```python
from build123d import *

# Parameters (mm, degrees)
BOSS_EXTRUDE1_DEPTH      = 20
BOSS_EXTRUDE1_DEPTH_BACK = 20
SKETCH1_W                = 35
SKETCH1_H                = 85.2
CUT_EXTRUDE2_REACH       = 91.478
SKETCH5_R                = 1.55
SKETCH5_R_2              = 2.9
CUT_EXTRUDE3_DEPTH       = 8
BOSS_EXTRUDE2_DEPTH      = 40


with BuildPart() as part:
    # Sketch1 → Boss-Extrude1 (new, two sides: drawn at the far end of the back side and taken through both)
    with BuildSketch(Plane.XY.offset(-BOSS_EXTRUDE1_DEPTH_BACK)):
        with Locations((1.938408795, -35.043181818)):
            Rectangle(SKETCH1_W, SKETCH1_H)
    extrude(amount=BOSS_EXTRUDE1_DEPTH + BOSS_EXTRUDE1_DEPTH_BACK)

    # Sketch2 → Cut-Extrude2 (cut, up to next)
    with BuildSketch(Plane.XY.offset(20), mode=Mode.PRIVATE) as cut_extrude2_sk1:
        with BuildLine():
            Line((-9.561591205, -10.793181818), (-9.561591205, -15.293181818))
            ThreePointArc((-9.561591205, -15.293181818), (-9.268697986, -16.000288599), (-8.561591205, -16.293181818))
            Line((-8.561591205, -16.293181818), (12.438408795, -16.293181818))
            ThreePointArc((12.438408795, -16.293181818), (13.145515577, -16.000288599), (13.438408795, -15.293181818))
            Line((13.438408795, -15.293181818), (13.438408795, -10.793181818))
            ThreePointArc((13.438408795, -10.793181818), (13.145515577, -10.086075037), (12.438408795, -9.793181818))
            Line((12.438408795, -9.793181818), (-8.561591205, -9.793181818))
            ThreePointArc((-8.561591205, -9.793181818), (-9.268697986, -10.086075037), (-9.561591205, -10.793181818))
        make_face()
    cut_extrude2_tool1 = extrude(cut_extrude2_sk1.sketch, amount=-CUT_EXTRUDE2_REACH, mode=Mode.PRIVATE) & part.part
    # Sketch2 → Cut-Extrude2 (cut, up to next)
    with BuildSketch(Plane.XY.offset(20), mode=Mode.PRIVATE) as cut_extrude2_sk2:
        with BuildLine():
            Line((-9.561591205, -21.793181818), (-9.561591205, -26.293181818))
            ThreePointArc((-9.561591205, -26.293181818), (-9.268697986, -27.000288599), (-8.561591205, -27.293181818))
            Line((-8.561591205, -27.293181818), (12.438408795, -27.293181818))
            ThreePointArc((12.438408795, -27.293181818), (13.145515577, -27.000288599), (13.438408795, -26.293181818))
            Line((13.438408795, -26.293181818), (13.438408795, -21.793181818))
            ThreePointArc((13.438408795, -21.793181818), (13.145515577, -21.086075037), (12.438408795, -20.793181818))
            Line((12.438408795, -20.793181818), (-8.561591205, -20.793181818))
            ThreePointArc((-8.561591205, -20.793181818), (-9.268697986, -21.086075037), (-9.561591205, -21.793181818))
        make_face()
    cut_extrude2_tool2 = extrude(cut_extrude2_sk2.sketch, amount=-CUT_EXTRUDE2_REACH, mode=Mode.PRIVATE) & part.part
    # Sketch2 → Cut-Extrude2 (cut, up to next)
    with BuildSketch(Plane.XY.offset(20), mode=Mode.PRIVATE) as cut_extrude2_sk3:
        with BuildLine():
            Line((-8.561591205, 1.206818182), (12.438408795, 1.206818182))
            ThreePointArc((12.438408795, 1.206818182), (13.145515577, 0.913924963), (13.438408795, 0.206818182))
            Line((13.438408795, 0.206818182), (13.438408795, -4.293181818))
            ThreePointArc((13.438408795, -4.293181818), (13.145515577, -5.000288599), (12.438408795, -5.293181818))
            Line((12.438408795, -5.293181818), (-8.561591205, -5.293181818))
            ThreePointArc((-8.561591205, -5.293181818), (-9.268697986, -5.000288599), (-9.561591205, -4.293181818))
            Line((-9.561591205, -4.293181818), (-9.561591205, 0.206818182))
            ThreePointArc((-9.561591205, 0.206818182), (-9.268697986, 0.913924963), (-8.561591205, 1.206818182))
        make_face()
    cut_extrude2_tool3 = extrude(cut_extrude2_sk3.sketch, amount=-CUT_EXTRUDE2_REACH, mode=Mode.PRIVATE) & part.part
    # Sketch2 → Cut-Extrude2 (cut, up to next)
    with BuildSketch(Plane.XY.offset(20), mode=Mode.PRIVATE) as cut_extrude2_sk4:
        with BuildLine():
            Line((-9.561591205, -32.793181818), (-9.561591205, -37.293181818))
            ThreePointArc((-9.561591205, -37.293181818), (-9.268697986, -38.000288599), (-8.561591205, -38.293181818))
            Line((-8.561591205, -38.293181818), (12.438408795, -38.293181818))
            ThreePointArc((12.438408795, -38.293181818), (13.145515577, -38.000288599), (13.438408795, -37.293181818))
            Line((13.438408795, -37.293181818), (13.438408795, -32.793181818))
            ThreePointArc((13.438408795, -32.793181818), (13.145515577, -32.086075037), (12.438408795, -31.793181818))
            Line((12.438408795, -31.793181818), (-8.561591205, -31.793181818))
            ThreePointArc((-8.561591205, -31.793181818), (-9.268697986, -32.086075037), (-9.561591205, -32.793181818))
        make_face()
    cut_extrude2_tool4 = extrude(cut_extrude2_sk4.sketch, amount=-CUT_EXTRUDE2_REACH, mode=Mode.PRIVATE) & part.part
    # Sketch2 → Cut-Extrude2 (cut, up to next)
    with BuildSketch(Plane.XY.offset(20), mode=Mode.PRIVATE) as cut_extrude2_sk5:
        with BuildLine():
            Line((-9.561591205, -43.793181818), (-9.561591205, -48.293181818))
            ThreePointArc((-9.561591205, -48.293181818), (-9.268697986, -49.000288599), (-8.561591205, -49.293181818))
            Line((-8.561591205, -49.293181818), (12.438408795, -49.293181818))
            ThreePointArc((12.438408795, -49.293181818), (13.145515577, -49.000288599), (13.438408795, -48.293181818))
            Line((13.438408795, -48.293181818), (13.438408795, -43.793181818))
            ThreePointArc((13.438408795, -43.793181818), (13.145515577, -43.086075037), (12.438408795, -42.793181818))
            Line((12.438408795, -42.793181818), (-8.561591205, -42.793181818))
            ThreePointArc((-8.561591205, -42.793181818), (-9.268697986, -43.086075037), (-9.561591205, -43.793181818))
        make_face()
    cut_extrude2_tool5 = extrude(cut_extrude2_sk5.sketch, amount=-CUT_EXTRUDE2_REACH, mode=Mode.PRIVATE) & part.part
    # Sketch2 → Cut-Extrude2 (cut, up to next)
    with BuildSketch(Plane.XY.offset(20), mode=Mode.PRIVATE) as cut_extrude2_sk6:
        with BuildLine():
            Line((-9.561591205, -54.793181818), (-9.561591205, -59.293181818))
            ThreePointArc((-9.561591205, -59.293181818), (-9.268697986, -60.000288599), (-8.561591205, -60.293181818))
            Line((-8.561591205, -60.293181818), (12.438408795, -60.293181818))
            ThreePointArc((12.438408795, -60.293181818), (13.145515577, -60.000288599), (13.438408795, -59.293181818))
            Line((13.438408795, -59.293181818), (13.438408795, -54.793181818))
            ThreePointArc((13.438408795, -54.793181818), (13.145515577, -54.086075037), (12.438408795, -53.793181818))
            Line((12.438408795, -53.793181818), (-8.561591205, -53.793181818))
            ThreePointArc((-8.561591205, -53.793181818), (-9.268697986, -54.086075037), (-9.561591205, -54.793181818))
        make_face()
    cut_extrude2_tool6 = extrude(cut_extrude2_sk6.sketch, amount=-CUT_EXTRUDE2_REACH, mode=Mode.PRIVATE) & part.part
    # Sketch2 → Cut-Extrude2 (cut, up to next)
    with BuildSketch(Plane.XY.offset(20), mode=Mode.PRIVATE) as cut_extrude2_sk7:
        with BuildLine():
            Line((-9.561591205, -65.793181818), (-9.561591205, -70.293181818))
            ThreePointArc((-9.561591205, -70.293181818), (-9.268697986, -71.000288599), (-8.561591205, -71.293181818))
            Line((-8.561591205, -71.293181818), (12.438408795, -71.293181818))
            ThreePointArc((12.438408795, -71.293181818), (13.145515577, -71.000288599), (13.438408795, -70.293181818))
            Line((13.438408795, -70.293181818), (13.438408795, -65.793181818))
            ThreePointArc((13.438408795, -65.793181818), (13.145515577, -65.086075037), (12.438408795, -64.793181818))
            Line((12.438408795, -64.793181818), (-8.561591205, -64.793181818))
            ThreePointArc((-8.561591205, -64.793181818), (-9.268697986, -65.086075037), (-9.561591205, -65.793181818))
        make_face()
    cut_extrude2_tool7 = extrude(cut_extrude2_sk7.sketch, amount=-CUT_EXTRUDE2_REACH, mode=Mode.PRIVATE) & part.part
    add(cut_extrude2_tool1.solids().sort_by_distance((1.938409, -13.043182, 20))[0], mode=Mode.SUBTRACT)
    add(cut_extrude2_tool2.solids().sort_by_distance((1.938409, -24.043182, 20))[0], mode=Mode.SUBTRACT)
    add(cut_extrude2_tool3.solids().sort_by_distance((1.938409, -2.043182, 20))[0], mode=Mode.SUBTRACT)
    add(cut_extrude2_tool4.solids().sort_by_distance((1.938409, -35.043182, 20))[0], mode=Mode.SUBTRACT)
    add(cut_extrude2_tool5.solids().sort_by_distance((1.938409, -46.043182, 20))[0], mode=Mode.SUBTRACT)
    add(cut_extrude2_tool6.solids().sort_by_distance((1.938409, -57.043182, 20))[0], mode=Mode.SUBTRACT)
    add(cut_extrude2_tool7.solids().sort_by_distance((1.938409, -68.043182, 20))[0], mode=Mode.SUBTRACT)

    # Sketch5 → Cut-Extrude3 (cut)
    with BuildSketch(Plane(origin=(0, 7.556818182, 0), x_dir=(1, 0, 0), z_dir=(0, 1, 0))):
        with Locations(Location((-3.046694012, 4.985102807, 0), (0, 0, 270))):
            Circle(SKETCH5_R)
        with Locations(Location((1.938408795, 0, 0), (0, 0, 270))):
            Circle(SKETCH5_R_2)
        with Locations(Location((6.923511603, 4.985102807, 0), (0, 0, 270))):
            Circle(SKETCH5_R)
        with Locations(Location((6.923511603, -4.985102807, 0), (0, 0, 270))):
            Circle(SKETCH5_R)
        with Locations(Location((-3.046694012, -4.985102807, 0), (0, 0, 270))):
            Circle(SKETCH5_R)
    cut_extrude3 = extrude(amount=-CUT_EXTRUDE3_DEPTH, mode=Mode.SUBTRACT)

    # Mirror3: Cut-Extrude3 across plane
    add(cut_extrude3.mirror(Plane.ZX.offset(-35.043181818)), mode=Mode.SUBTRACT)

    # Sketch7 → Boss-Extrude2 (add)
    with BuildSketch(Plane(origin=(0, 0, -20), x_dir=(-1, 0, 0), z_dir=(0, 0, -1))):
        with BuildLine():
            Line((-19.438408795, 7.556818182), (-21.818320385, 7.556818182))
            ThreePointArc((-21.818320385, 7.556818182), (-23.528170709, 6.594320889), (-23.592294725, 4.633230049))
            Line((-23.592294725, 4.633230049), (-20.794562752, -0.740490723))
            ThreePointArc((-20.794562752, -0.740490723), (-19.782377041, -3.429490161), (-19.438408795, -6.282019519))
            Line((-19.438408795, -6.282019519), (-19.438408795, 7.556818182))
        make_face()
        with BuildLine():
            Line((15.561591205, -77.643181818), (17.941502794, -77.643181818))
            ThreePointArc((17.941502794, -77.643181818), (19.651353118, -76.680684525), (19.715477134, -74.719593686))
            Line((19.715477134, -74.719593686), (16.917745161, -69.345872913))
            ThreePointArc((16.917745161, -69.345872913), (15.90555945, -66.656873475), (15.561591205, -63.804344117))
            Line((15.561591205, -63.804344117), (15.561591205, -77.643181818))
        make_face()
        with BuildLine():
            Line((-19.438408795, -63.804344117), (-19.438408795, -77.643181818))
            Line((-19.438408795, -77.643181818), (-21.818320385, -77.643181818))
            ThreePointArc((-21.818320385, -77.643181818), (-23.528170709, -76.680684525), (-23.592294725, -74.719593686))
            Line((-23.592294725, -74.719593686), (-20.794562752, -69.345872913))
            ThreePointArc((-20.794562752, -69.345872913), (-19.782377041, -66.656873475), (-19.438408795, -63.804344117))
        make_face()
        with BuildLine():
            Line((15.561591205, -6.282019519), (15.561591205, 7.556818182))
            Line((15.561591205, 7.556818182), (17.941502794, 7.556818182))
            ThreePointArc((17.941502794, 7.556818182), (19.651353118, 6.594320889), (19.715477134, 4.633230049))
            Line((19.715477134, 4.633230049), (16.917745161, -0.740490723))
            ThreePointArc((16.917745161, -0.740490723), (15.90555945, -3.429490161), (15.561591205, -6.282019519))
        make_face()
    extrude(amount=-BOSS_EXTRUDE2_DEPTH)


solid = part.part
```
Model file for the job. Use its own axes, mm. A direction names the side the tool comes from. Coordinates: 2 decimals unless noted, no trailing zeros. Order: outer loops, then holes, each group sorted by start corner. A loop starts at its lowest first (then second) coordinate and runs counter-clockwise, first axis right, second up. Notation, with made-up numbers: (44, 49.25) -> (74, 49.25) arc R21 cw to (74, 82.25) -> close; hole circle Ø10 at (-36, 57.5). An arc over 180 degrees is marked (long way). Return JSON: item names as keys, results as strings.
Item 1: 3-axis set-ups, long thin cutter, end or side, ignore diameter. For faces 1 (the face through (-15.915, -3.39, -0.28)), 2 (the face through (7.389, -74.513, 6.464)), 3 (the face through (-9.562, -35, 0)), 4 (the face through (7.389, 4.426, 6.464)): which of +Z, -Z, +X, -X, +Y, -Y reach the whole face in a straight line?
Model answer:
{"face 1": "+Z, -Z, -X", "face 2": "-Y", "face 3": "+Z, -Z", "face 4": "+Y"}
Item 2: Mould opens along X. For faces 5 (the face through (-15.915, -66.696, -0.28)), 6 (the face through (-9.562, -46, 0)), 7 (the face through (23.51, -76.71, -0.28)) say: pulls with the +X half, pulls with the -X half, needs draft (parallel to the pull), parting line crosses it, or undercut.
Model answer:
{"face 5": "pulls with the -X half", "face 6": "undercut", "face 7": "pulls with the +X half"}
Item 3: Pin check, flat tips, straight feed: P1, Ø3.5, axis at y = -46.5, z = 5.5, coming from the -X side; P2, Ø3, axis at x = -3.05, z = -4.99, coming from the -Y side; P3, Ø4, axis at x = 5, y = -1.5, coming from the +Z side; P4, Ø2.5, axis at x = 6.92, z = -4.99, coming from the +Y side. Stop position of each tip, or through.
Model answer:
{"P1": "stops at x = -15.56", "P2": "stops at y = -64.79", "P3": "passes through", "P4": "stops at y = -5.29"}
Item 4: Slice it at D-D (y = -52.5). Write the cut outline in (x, z), then the cut area to 3 significant figures.
Model answer:
{"outline": "(-15.56, -20) -> (19.44, -20) -> (19.44, 20) -> (-15.56, 20) -> close", "area": "1,400 mm²"}
Item 5: Slice it at A-A (y = -24). Write the cut outline in (x, z).
Model answer:
{"outline": "(-15.56, -20) -> (-9.56, -20) -> (-9.56, 20) -> (-15.56, 20) -> close; (13.44, -20) -> (19.44, -20) -> (19.44, 20) -> (13.44, 20) -> close"}
Item 6: Wall check: line 1 along X through (y, z) = (-25, -16); line 2 along X through (y, z) = (3.5, 1); line 3 along X through (y, z) = (-39, -11). Give the ranges that are in metal, low to high. Write a range as from..to.
Model answer:
{"line 1": "x = -15.56..-9.56, 13.44..19.44", "line 2": "x = -19.13..-0.78, 4.66..23", "line 3": "x = -15.56..19.44"}
Item 7: Slice it at B-B (x = 10.5). Count the separate pieces of the cut face and the enclosed holes in it, then the cut area to 3 significant figures.
Model answer:
{"separate pieces": "8", "enclosed holes": "0", "area": "1,590 mm²"}
